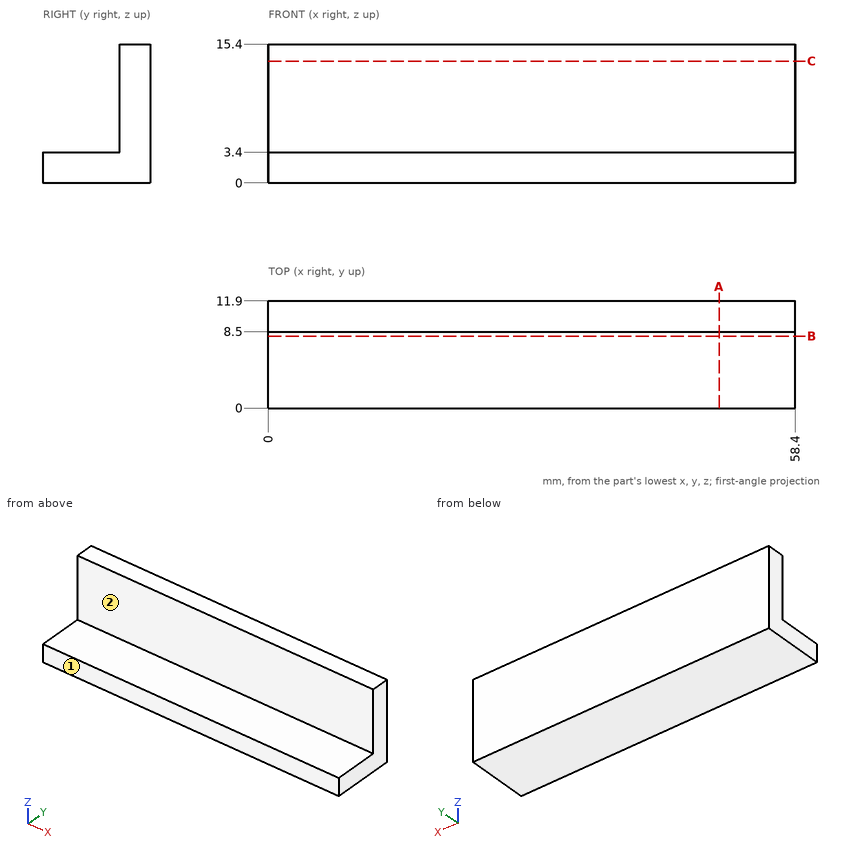
The figure shows three views and two pictorial views of one solid part (mm, origin at its lowest corner). Answer the questions. A direction names the side the tool comes from. Coordinates: 2 decimals unless noted, no trailing zeros. Loops run counter-clockwise (first coordinate to the right, second up) from the corner with the lowest first, then second, coordinate; pieces in that order, holes last.
1) Find section A-A on x = 50. Write down the section's boundary in (y, z), then the cut area to 3 significant figures.
2) A flat-ended cylindrical pin translates along its axis: pin 1 Ø1.5 at (x, z) = (39, 5) entering from -Y. Find the tip coordinate at first contact, or state that the pin passes through.
3) Find the intervals of material crossed by L1, parallel to Z at x = 18, y = 8; L2, parallel to Y at x = 16.5, z = 9.25, in increasing order.
4) A tool of negligible diameter and unlimited length cuts with its end or side. For the marked faces 1 and 2, from which of +Z, -Z, +X, -X, +Y, -Y can it reach the whole face along a straight path? Write none if from no direction.
5) Find section B-B on y = 8. Write down the section's boundary in (x, z).
6) Find section C-C on z = 13.5. Write down the section's boundary in (x, y).
Values:
1. outline: (0, 0) - (11.9, 0) - (11.9, 15.4) - (8.5, 15.4) - (8.5, 3.4) - (0, 3.4) - close
1. area: 81.3 mm2
2. pin 1: stops at y = 8.5
3. L1: z = 0 to 3.4
3. L2: y = 8.5 to 11.9
4. face 1: +Z, -Z, +X, -X, -Y
4. face 2: +Z, +X, -X, -Y
5. outline: (0, 0) - (58.4, 0) - (58.4, 3.4) - (0, 3.4) - close
6. outline: (0, 8.5) - (58.4, 8.5) - (58.4, 11.9) - (0, 11.9) - close
